Check sheet for the modelled part. Datum: model origin and axes. Units: mm. Face numbers are marked on the shaded views. Give positions to 0.01 mm unless a question says otherwise; leave off trailing zeros. Loops run counter-clockwise (first coordinate to the right, second up) from the corner with the lowest first, then second, coordinate; pieces in that order, holes last. Notation, with made-up numbers: M -21,-33.75 L 36,-33.75 A9 cw 36,-16.75 Z; hole C -39,48.5 d9. An arc over 180 degrees is marked long. One line per question, with ' | ' between items. Start each with the question number.
from build123d import *

# Parameters (mm, degrees)
SKETCH_W  = 35
SKETCH_H  = 30
SKETCH_R  = 3
PAD_DEPTH = 10
FILLET_R  = 2


with BuildPart() as part:
    # Sketch → Pad (new body)
    with BuildSketch(Plane.XY):
        Rectangle(SKETCH_W, SKETCH_H)
        with Locations((-13, 10)):
            Circle(SKETCH_R, mode=Mode.SUBTRACT)
        with Locations((13, 10)):
            Circle(SKETCH_R, mode=Mode.SUBTRACT)
        with Locations((13, -10)):
            Circle(SKETCH_R, mode=Mode.SUBTRACT)
        with Locations((-13, -10)):
            Circle(SKETCH_R, mode=Mode.SUBTRACT)
    extrude(amount=PAD_DEPTH)

    # Fillet
    fillet_edges = [part.edges().sort_by_distance(p)[0] for p in [
        (-17.5, -15, 5),
        (17.5, -15, 5),
        (17.5, 15, 5),
        (-17.5, 15, 5),
    ]]
    fillet(fillet_edges, radius=FILLET_R)


solid = part.part
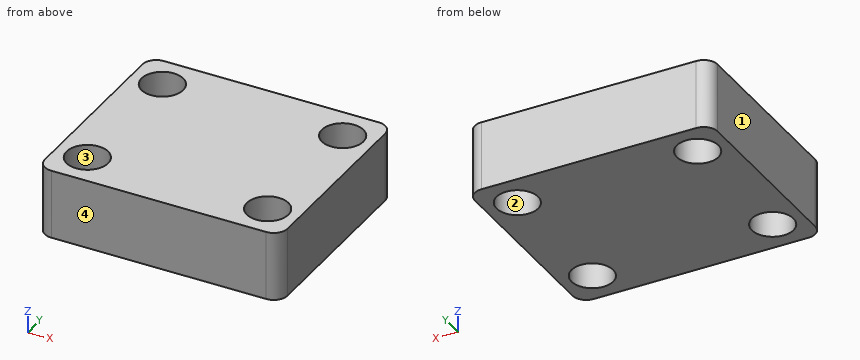
Q1. Material ranges on probe 1 along Y at (x, z) = (13, 6.5); probe 2 along X at (y, z) = (-12.25, 0.5); probe 3 along Y at (x, z) = (15, 6.25), recorded low to high. Write a range as from..to.
Q2. Cross-section at A-A (z = 6). Record the cut outline in (x, y).
Q3. Cross-section at C-C (x = -13). Record the cut outline in (y, z), and give its area (3 significant figures).
Q4. Cross-section at B-B (y = -10). Record the cut outline in (x, z), and give its area (3 significant figures).
Q5. Draft check along X on the marked faces 1, 2, 3 and 4. Enter one of: released by +X, released by -X, zero draft, split by the parting line, or undercut.
Solved:
1) probe 1: y = -15..-13, -7..7, 13..15 | probe 2: x = -17.5..-14.98, -11.02..11.02, 14.98..17.5 | probe 3: y = -15..-12.24, -7.76..7.76, 12.24..15
2) outline: M -17.5,-13 A2 ccw -15.5,-15 L 15.5,-15 A2 ccw 17.5,-13 L 17.5,13 A2 ccw 15.5,15 L -15.5,15 A2 ccw -17.5,13 Z; hole C -13,-10 d6; hole C -13,10 d6; hole C 13,-10 d6; hole C 13,10 d6
3) outline: M -15,0 L -13,0 L -13,10 L -15,10 Z; M -7,0 L 7,0 L 7,10 L -7,10 Z; M 13,0 L 15,0 L 15,10 L 13,10 Z | area: 180 mm²
4) outline: M -17.5,0 L -16,0 L -16,10 L -17.5,10 Z; M -10,0 L 10,0 L 10,10 L -10,10 Z; M 16,0 L 17.5,0 L 17.5,10 L 16,10 Z | area: 230 mm²
5) face 1: released by -X | face 2: undercut | face 3: undercut | face 4: zero draft
